Input: part model. Units: mm. Frame: model coordinates. A direction names the side the tool comes from. Give positions to 0.01 mm unless a question says otherwise; leave off trailing zeros. Loops run counter-clockwise (first coordinate to the right, second up) from the corner with the lowest first, then second, coordinate; pieces in that order, holes last. Notation, with made-up numbers: (35.25, 4.5) -> (72.25, 4.5) arc R26 ccw to (72.25, 37.5) -> close; hole circle Ø5 at (78, 80). An arc over 180 degrees is marked (long way). Answer as a JSON object with one key per item and string values.
```python
from build123d import *
from build123d.topology import SkipClean

# Parameters (mm, degrees)
BOSS_EXTRU_1_START      = -6
BOSS_EXTRU_1_DEPTH      = 6
BOSS_EXTRU_2_START      = -6
BOSS_EXTRU_2_DEPTH      = 2
ENL_V_START             = -4
ENL_V_MAT_EXTRU_1_DEPTH = 4
ENL_V_START_2           = -16.5
ENL_V_MAT_EXTRU_5_DEPTH = 10.5
CONG_1_R                = 2
CHANFREIN1_SIZE         = 0.5
SYM_TRIE1_START         = -2
SYM_TRIE1_DEPTH         = 10.5
SYM_TRIE1_START_2       = -8
SYM_TRIE1_2_DEPTH       = 4
SYM_TRIE1_START_3       = -7.5000001
SYM_TRIE1_3_DEPTH       = 5.5000001
SYM_TRIE1_START_4       = -4
SYM_TRIE1_4_DEPTH       = 2
SYM_TRIE1_7_DEPTH       = 0.4999999
M3_CLEARANCE_HOLE1_D    = 3.4
BOSS_EXTRU_3_DEPTH      = 8.5
ENL_V_START_3           = -8.5
ENL_V_MAT_EXTRU_2_DEPTH = 8.5
ENL_V_START_4           = -6.5
ESQUISSE5_R             = 1.125
ENL_V_MAT_EXTRU_3_DEPTH = 6
ESQUISSE5_3_R           = 1.125
ENL_V_MAT_EXTRU_4_DEPTH = 6.5
CONG_2_R                = 0.5
CONG_3_R                = 1.5
ENL_V_START_5           = -7.5
ESQUISSE9_R             = 4
ENL_V_MAT_EXTRU_8_DEPTH = 7.5
CONG_5_R                = 1.5
CHANFREIN2_SIZE         = 1


with BuildPart() as part:
    # Esquisse1 → Révolution1 (revolve)
    with BuildSketch(Plane.XY):
        Polygon((-8.5, 8.5), (-6, 8.5), (-6, 0), (-3.5, 0), (-3.5, -1), (-4.383974596, -1), (-5.25, -1.5), (-6.5, -1.5), (-6.5, -8), (-8.5, -8), align=None)
    revolve(axis=Axis((0, 6.43509573, 0), (0, -1, 0)))

    # Esquisse3 → Boss.-Extru.1 (add)
    with BuildSketch(Plane.XZ.offset(8).offset(BOSS_EXTRU_1_START)):
        with BuildLine():
            ThreePointArc((-7.928571429, 3.06394437), (-7.728470361, 3.5384666), (-7.5, 4))
            Line((-7.5, 4), (-10.5, 4))
            ThreePointArc((-10.5, 4), (-14.5, 0), (-10.5, -4))
            Line((-10.5, -4), (-7.5, -4))
            ThreePointArc((-7.5, -4), (-7.728470361, -3.5384666), (-7.928571429, -3.06394437))
            ThreePointArc((-7.928571429, -3.06394437), (-8.196108254, -2.252511816), (-8.380833333, -1.418320358))
            ThreePointArc((-8.380833333, -1.418320358), (-13.05, 0), (-8.380833333, 1.418320358))
            ThreePointArc((-8.380833333, 1.418320358), (-8.196108254, 2.252511816), (-7.928571429, 3.06394437))
        make_face()
    extrude(amount=BOSS_EXTRU_1_DEPTH)

    # Esquisse3<4> → Boss.-Extru.2 (add)
    with BuildSketch(Plane.XZ.offset(8).offset(BOSS_EXTRU_2_START)):
        with BuildLine():
            ThreePointArc((-8.380833333, -1.418320358), (-8.5, 0), (-8.380833333, 1.418320358))
            ThreePointArc((-8.380833333, 1.418320358), (-13.05, 0), (-8.380833333, -1.418320358))
        make_face()
    extrude(amount=BOSS_EXTRU_2_DEPTH)

    # Esquisse3<5> → Enlèv. mat.-Extru.1 (cut)
    with SkipClean():  # the faces are left unmerged after this step: merging them gives an invalid solid
        with BuildSketch(Plane.XZ.offset(8).offset(ENL_V_START)):
            with BuildLine():
                ThreePointArc((-7.95, 0), (-8.06008453, 0.741156191), (-8.380833333, 1.418320358))
                ThreePointArc((-8.380833333, 1.418320358), (-8.5, 0), (-8.380833333, -1.418320358))
                ThreePointArc((-8.380833333, -1.418320358), (-8.06008453, -0.741156191), (-7.95, 0))
            make_face()
        extrude(amount=ENL_V_MAT_EXTRU_1_DEPTH, mode=Mode.SUBTRACT)

    # Esquisse3<7> → Enlèv. mat.-Extru.5 (cut)
    with SkipClean():  # the faces are left unmerged after this step: merging them gives an invalid solid
        with BuildSketch(Plane.XZ.offset(8).offset(ENL_V_START_2)):
            with BuildLine():
                ThreePointArc((-7.5, 4), (-8.5, 0), (-7.5, -4))
                Line((-7.5, -4), (-7.5, 4))
            make_face()
        extrude(amount=ENL_V_MAT_EXTRU_5_DEPTH, mode=Mode.SUBTRACT)

    # Congé1
    # the kernel refuses this fillet: 2 mm, written as the material it adds along each edge
    with BuildSketch(Plane(origin=(-7.5, -2, 4), x_dir=(0.5219209843200922, 0, 0.8529938370975175), z_dir=(0, -1, 0))) as cong_1_piece_1:
        with BuildLine():
            CenterArc((1.12308337, 1.996502992), CONG_1_R, 211.461195757, 55.150095421)
            Line((-0.582904304, 0.952661023), (0, 0))
            ThreePointArc((0, 0), (0.502432034, 0.014862284), (1.004864068, 0))
        make_face()
    extrude(amount=6)
    with BuildSketch(Plane(origin=(-7.5, -2, -4), x_dir=(0.521920984320094, 0, -0.8529938370975163), z_dir=(0, -1, 0))) as cong_1_piece_2:
        with BuildLine():
            CenterArc((1.12308337, -1.996502992), CONG_1_R, 93.388708822, 55.150095421)
            Line((-0.582904304, -0.952661023), (0, 0))
            ThreePointArc((0, 0), (0.502432034, -0.014862284), (1.004864068, 0))
        make_face()
    extrude(amount=6)

    # Chanfrein1
    chanfrein1_edges = [part.edges().sort_by_distance(p)[0] for p in [
        (-7.95, -8, 0),
    ]]
    chamfer(chanfrein1_edges, length=CHANFREIN1_SIZE)

    # Symétrie1: read off the stored shape, not the designer's step
    # Symétrie1 outline → Symétrie1 (cut)
    with BuildSketch(Plane(origin=(0, 0, 0), x_dir=(1, 0, 0), z_dir=(0, 1, 0)).offset(SYM_TRIE1_START)):
        with BuildLine():
            Line((7.5, 4), (7.5, -4))
            ThreePointArc((7.5, -4), (8.5, 0), (7.5, 4))
        make_face()
    extrude(amount=SYM_TRIE1_DEPTH, mode=Mode.SUBTRACT)

    # Sym_trie1 2 outline → Sym_trie1 2 (cut)
    with BuildSketch(Plane(origin=(0, 0, 0), x_dir=(1, 0, 0), z_dir=(0, 1, 0)).offset(SYM_TRIE1_START_2)):
        with BuildLine():
            ThreePointArc((8.380833333, 1.418320358), (7.95, 0), (8.380833333, -1.418320358))
            ThreePointArc((8.380833333, -1.418320358), (8.5, 0), (8.380833333, 1.418320358))
        make_face()
    extrude(amount=SYM_TRIE1_2_DEPTH, mode=Mode.SUBTRACT)

    # Sym_trie1 3 outline → Sym_trie1 3 (add)
    with BuildSketch(Plane(origin=(0, 0, 0), x_dir=(1, 0, 0), z_dir=(0, 1, 0)).offset(SYM_TRIE1_START_3)):
        with BuildLine():
            ThreePointArc((6.975540357, -4.857142857), (7.69102387, -4.227189479), (8.61684397, -4))
            Line((8.61684397, -4), (10.5, -4))
            ThreePointArc((10.5, -4), (14.5, 0), (10.5, 4))
            Line((10.5, 4), (8.61684397, 4))
            ThreePointArc((8.61684397, 4), (7.69102387, 4.227189479), (6.975540357, 4.857142857))
            ThreePointArc((6.975540357, 4.857142857), (7.868349781, 3.215442696), (8.380833333, 1.418320358))
            ThreePointArc((8.380833333, 1.418320358), (13.05, 0), (8.380833333, -1.418320358))
            ThreePointArc((8.380833333, -1.418320358), (7.868349781, -3.215442696), (6.975540357, -4.857142857))
        make_face()
    extrude(amount=SYM_TRIE1_3_DEPTH)

    # Sym_trie1 4 outline → Sym_trie1 4 (add)
    with BuildSketch(Plane(origin=(0, 0, 0), x_dir=(1, 0, 0), z_dir=(0, 1, 0)).offset(SYM_TRIE1_START_4)):
        with BuildLine():
            ThreePointArc((8.380833333, 1.418320358), (8.5, 0), (8.380833333, -1.418320358))
            ThreePointArc((8.380833333, -1.418320358), (13.05, 0), (8.380833333, 1.418320358))
        make_face()
    extrude(amount=SYM_TRIE1_4_DEPTH)

    # Sym_trie1 5 outline → Sym_trie1 5 (revolve, cut)
    with BuildSketch(Plane(origin=(10.5, 0, 0), x_dir=(1, 0, 0), z_dir=(0, 0, 1))):
        Polygon((3.05, -8), (2.55, -7.5), (2.55, -8), align=None)
    revolve(axis=Axis((10.5, 0, 0), (0, 1, 0)), mode=Mode.SUBTRACT)

    # Sym_trie1 6 outline → Sym_trie1 6 (revolve)
    with SkipClean():  # the faces are left unmerged after this step: merging them gives an invalid solid
        with BuildSketch(Plane(origin=(10.5, 0, 0), x_dir=(1, 0, 0), z_dir=(0, 0, 1))):
            Polygon((3.05, -7.5), (2.55, -7.5), (3.05, -8), align=None)
        revolve(axis=Axis((10.5, 0, 0), (0, 1, 0)))

    # Sym_trie1 7 outline → Sym_trie1 7 (add)
    with BuildSketch(Plane(origin=(0, 0, 0), x_dir=(1, 0, 0), z_dir=(0, 1, 0)).offset(SYM_TRIE1_START_2)):
        with BuildLine():
            ThreePointArc((8.2475, 2.056390953), (13.55, 0), (8.2475, -2.056390953))
            ThreePointArc((8.2475, -2.056390953), (7.933495012, -3.051173035), (7.5, -4))
            ThreePointArc((7.5, -4), (7.250447615, -4.436328367), (6.975540357, -4.857142857))
            ThreePointArc((6.975540357, -4.857142857), (7.69102387, -4.227189479), (8.61684397, -4))
            Line((8.61684397, -4), (10.5, -4))
            ThreePointArc((10.5, -4), (14.5, 0), (10.5, 4))
            Line((10.5, 4), (8.61684397, 4))
            ThreePointArc((8.61684397, 4), (7.69102387, 4.227189479), (6.975540357, 4.857142857))
            ThreePointArc((6.975540357, 4.857142857), (7.250447615, 4.436328367), (7.5, 4))
            ThreePointArc((7.5, 4), (7.933495012, 3.051173035), (8.2475, 2.056390953))
        make_face()
    extrude(amount=SYM_TRIE1_7_DEPTH)

    # M3 Clearance Hole1 (through all)
    with Locations(Plane(origin=(0, -4, 0), x_dir=(-1, 0, 0), z_dir=(0, -1, 0))):
        with Locations((10.5, 0), (-10.5, 0)):
            Hole(M3_CLEARANCE_HOLE1_D / 2)

    # Esquisse4 → Boss.-Extru.3 (add)
    with BuildSketch(Plane(origin=(0, 8.5, 0), x_dir=(1, 0, 0), z_dir=(0, 1, 0))):
        with BuildLine():
            Line((7.5, 14.5), (-7.5, 14.5))
            Line((-7.5, 14.5), (-7.5, 4))
            ThreePointArc((-7.5, 4), (-1.593272922, 8.349340177), (5.5, 6.480740698))
            Line((5.5, 6.480740698), (5.5, 13))
            Line((5.5, 13), (6, 13))
            Line((6, 13), (6, 6.020797289))
            ThreePointArc((6, 6.020797289), (6.825203691, 5.066220937), (7.5, 4))
            Line((7.5, 4), (7.5, 14.5))
        make_face()
    extrude(amount=-BOSS_EXTRU_3_DEPTH)

    # Esquisse4<3> → Enlèv. mat.-Extru.2 (cut)
    with BuildSketch(Plane(origin=(0, 8.5, 0), x_dir=(1, 0, 0), z_dir=(0, 1, 0)).offset(ENL_V_START_3)):
        with BuildLine():
            Line((6, 0), (6, 13))
            Line((6, 13), (5.5, 13))
            Line((5.5, 13), (5.5, 2.397915762))
            ThreePointArc((5.5, 2.397915762), (5.873670062, 1.224744871), (6, 0))
        make_face()
    extrude(amount=ENL_V_MAT_EXTRU_2_DEPTH, mode=Mode.SUBTRACT)

    # Esquisse5 → Enlèv. mat.-Extru.3 (cut)
    with BuildSketch(Plane(origin=(7.5, 0, 0), x_dir=(0, 0, -1), z_dir=(1, 0, 0)).offset(ENL_V_START_4)):
        with Locations((9.875, 4.2554)):
            Circle(ESQUISSE5_R)
        with BuildLine():
            Line((8.75, 8.5), (8.75, 4.2554))
            ThreePointArc((8.75, 4.2554), (9.875, 5.3804), (11, 4.2554))
            Line((11, 4.2554), (11, 8.5))
            Line((11, 8.5), (8.75, 8.5))
        make_face()
    extrude(amount=-ENL_V_MAT_EXTRU_3_DEPTH, mode=Mode.SUBTRACT)

    # Esquisse5<3> → Enlèv. mat.-Extru.4 (cut)
    with BuildSketch(Plane(origin=(7.5, 0, 0), x_dir=(0, 0, -1), z_dir=(1, 0, 0))):
        with Locations(Location((9.875, 4.2554, 0), (0, 0, 180))):
            Circle(ESQUISSE5_3_R)
    extrude(amount=-ENL_V_MAT_EXTRU_4_DEPTH, mode=Mode.SUBTRACT)

    # Congé2
    # the kernel refuses this fillet: 0.5 mm, written as the material it takes off along each edge
    with BuildSketch(Plane(origin=(5.5, 0, -2.397915762), x_dir=(0, 0, -1), z_dir=(0, 1, 0))) as cong_2_piece_1:
        with BuildLine():
            CenterArc((1.75539617, 0.5), CONG_2_R, 129.715137232, 140.284862768)
            ThreePointArc((1.435910637, 0.884615385), (0.749192225, 0.391603841), (0, 0))
            Line((0, 0), (1.75539617, 0))
        make_face()
    extrude(amount=12.888490425, mode=Mode.SUBTRACT)

    # Congé3
    cong_3_edges = [part.edges().sort_by_distance(p)[0] for p in [
        (7.5, 3.25, 4),
        (7.5, 4.25, -14.5),
        (-7.5, 4.25, -14.5),
        (-7.5, 3.25, 4),
    ]]
    fillet(cong_3_edges, radius=CONG_3_R)

    # Esquisse9 → Enlèv. mat.-Extru.8 (cut)
    with BuildSketch(Plane(origin=(0, 8.5, 0), x_dir=(1, 0, 0), z_dir=(0, 1, 0)).offset(ENL_V_START_5)):
        with Locations((-10.5, 0)):
            Circle(ESQUISSE9_R)
        with Locations((10.5, 0)):
            Circle(ESQUISSE9_R)
    extrude(amount=ENL_V_MAT_EXTRU_8_DEPTH, mode=Mode.SUBTRACT)

    # Congé5
    cong_5_edges = [part.edges().sort_by_distance(p)[0] for p in [
        (7.5, 4.75, -2.645751311),
        (7.5, 4.75, 2.645751311),
        (-7.5, 4.75, -2.645751311),
        (-7.5, 4.75, 2.645751311),
    ]]
    fillet(cong_5_edges, radius=CONG_5_R)

    # Chanfrein2
    # the kernel refuses this chamfer: 1 mm, written as the material it takes off along each edge
    with BuildSketch(Plane(origin=(0, -8, 0), x_dir=(-1, 0, 0), z_dir=(0, 0, 1))) as chanfrein2_piece_1:
        Polygon((6.5 + CHANFREIN2_SIZE, 0), (6.5, -CHANFREIN2_SIZE), (6.5, 0), align=None)
    revolve(axis=Axis((0, -8, 0), (0, -1, 0)), mode=Mode.SUBTRACT)


solid = part.part
```
Q1. Pin query (flat end, axial travel): pin 1 (5.5 mm diameter, centred on x = 10.5, z = 0, fed in from +Y); pin 2 (4 mm diameter, centred on x = -10.5, z = 0, fed in from -Y); pin 3 (6 mm diameter, centred on x = -1, y = -4, fed in from -Z); pin 4 (2.5 mm diameter, centred on x = -10.5, z = 0, fed in from +Y) (3 decimals). Return the tip coordinate at first contact, or that it passes through.
Evaluation:
{"pin 1": "stops at y = -2", "pin 2": "stops at y = -4", "pin 3": "stops at z = -8.5", "pin 4": "passes through"}
Q2. Section C-C, the plane y = 6.5. Return the cut outline in (x, z).
Evaluation:
{"outline": "(-7.5, -13) arc R1.5 ccw to (-6, -14.5) -> (6, -14.5) arc R1.5 ccw to (7.5, -13) -> (7.5, -3.16) arc R1.5 ccw to (7.23, -2.3) arc R4 cw to (7.23, 2.3) arc R1.5 ccw to (7.5, 3.16) -> (7.5, 3.61) arc R1.5 ccw to (7.29, 4.38) arc R8.5 ccw to (-7.29, 4.38) arc R1.5 ccw to (-7.5, 3.61) -> (-7.5, 3.16) arc R1.5 ccw to (-7.23, 2.3) arc R4 cw to (-7.23, -2.3) arc R1.5 ccw to (-7.5, -3.16) -> close; hole (-5, -11) -> (1, -11) -> (1, -8.75) -> (-5, -8.75) -> close; hole (4.62, -3.83) arc R0.5 cw to (5.5, -4.15) -> (5.5, -13) -> (6, -13) -> (6, 0) arc R6 ccw (long way) to start"}
Q3. Access query for faces 1 (the cylindrical face through (-7.432, 4.698, -2.716)), 2 (the cylindrical face through (6.5, 4.7, 0)), 3 (the flat face through (-7.5, 3, -7)), 4 (the flat face through (-10, -5, 4)), 5 (the flat face through (-10, -4, -2)). Directions: +Z, -Z, +X, -X, +Y, -Y. A direction counts if a zero-diameter tool reaches every point of the face in a straight line with its end or side. Return the directions, or none.
Evaluation:
{"face 1": "-X, +Y", "face 2": "+X, +Y", "face 3": "+Z, -Z, -X, +Y", "face 4": "+Z, -X, +Y, -Y", "face 5": "-Y"}
Q4. Section D-D, the plane x = 1.75. Give the number of separate pieces and of enclosed holes in the cut face, then the cut area to 3 significant figures.
Evaluation:
{"separate pieces": "2", "enclosed holes": "1", "area": "133 mm2"}
Q5. Section B-B, the plane y = -5. Return the cut outline in (x, z).
Evaluation:
{"outline": "(-10.5, -4) -> (-8.62, -4) arc R2 cw to (-6.98, -4.86) arc R8.5 ccw to (6.98, -4.86) arc R2 cw to (8.62, -4) -> (10.5, -4) arc R4 ccw to (10.5, 4) -> (8.62, 4) arc R2 cw to (6.98, 4.86) arc R8.5 ccw to (-6.98, 4.86) arc R2 cw to (-8.62, 4) -> (-10.5, 4) arc R4 ccw to start; hole circle Ø5.1 at (-10.5, 0); hole circle Ø13 at (0, 0); hole circle Ø5.1 at (10.5, 0)"}
Q6. Ray query, line 1 along Z through (x, y) = (0, 6); line 2 along Z through (x, y) = (-1.75, 5.75); line 3 along Z through (x, y) = (10.5, -3.4). Return the intervals inside material, ascending.
Evaluation:
{"line 1": "z = -14.5 to -11, -8.75 to -6, 6 to 8.5", "line 2": "z = -14.5 to -11, -8.75 to -5.74, 5.74 to 8.32", "line 3": "z = -4 to -1.7, 1.7 to 4"}
Q7. Section A-A, the plane z = -12. Return the cut outline in (x, y).
Evaluation:
{"outline": "(-7.5, 0) -> (5.5, 0) -> (5.5, 8.5) -> (-7.5, 8.5) -> close; (6, 0) -> (7.5, 0) -> (7.5, 8.5) -> (6, 8.5) -> close"}
Q8. Draft query along Z for faces 6 (the flat face through (0, -1, 4)), 7 (the flat face through (7.5, 3, -6)), 8 (the flat face through (10, -5, -4)). Return one class per face: +Z half, -Z half, draft (parallel to the pull), parting line (faces both ways), or undercut.
Evaluation:
{"face 6": "undercut", "face 7": "draft", "face 8": "-Z half"}
